```python
from build123d import *

# Parameters (mm, degrees)
BOSS_EXTRUDE1_DEPTH = 28.575
CHAMFER1_SIZE       = 6.35
SKETCH3_R           = 1.905
CUT_EXTRUDE1_DEPTH  = 62.321512782
FILLET1_R           = 3.175
CUT_EXTRUDE4_START  = -6.35
CUT_EXTRUDE4_DEPTH  = 6.35
FILLET3_R           = 1.5875
FILLET5_R           = 1.5875


with BuildPart() as part:
    # Sketch2 → Boss-Extrude1 (new body)
    with BuildSketch(Plane.XY):
        with BuildLine():
            Line((0, 0), (19.056686619, 0))
            ThreePointArc((19.056686619, 0), (7.311521051, 25.4), (19.056686619, 50.8))
            Line((19.056686619, 50.8), (0, 50.8))
            Line((0, 50.8), (0, 0))
        make_face()
    extrude(amount=BOSS_EXTRUDE1_DEPTH)

    # Chamfer1
    chamfer1_edges = [part.edges().sort_by_distance(p)[0] for p in [
        (0, 0, 14.2875),
    ]]
    chamfer(chamfer1_edges, length=CHAMFER1_SIZE)

    # Sketch3 → Cut-Extrude1 (cut, through all)
    with BuildSketch(Plane.XY.offset(28.575)):
        with Locations((5.55625, 45.24375)):
            Circle(SKETCH3_R)
        with Locations((5.55625, 8.651474106)):
            Circle(SKETCH3_R)
    extrude(amount=-CUT_EXTRUDE1_DEPTH, mode=Mode.SUBTRACT)

    # Fillet1
    fillet1_edges = [part.edges().sort_by_distance(p)[0] for p in [
        (0, 50.8, 14.2875),
        (6.35, 0, 14.2875),
        (0, 6.35, 14.2875),
    ]]
    fillet(fillet1_edges, radius=FILLET1_R)

    # Sketch6 → Cut-Extrude4 (cut)
    with BuildSketch(Plane.XY.offset(28.575).offset(CUT_EXTRUDE4_START)):
        with BuildLine():
            Line((5.55625, 49.2125), (17.317631251, 49.2125))
            ThreePointArc((17.317631251, 49.2125), (14.028288765, 45.468022294), (11.333951868, 41.275))
            Line((11.333951868, 41.275), (5.55625, 41.275))
            ThreePointArc((5.55625, 41.275), (1.5875, 45.24375), (5.55625, 49.2125))
        make_face()
        with BuildLine():
            Line((5.55625, 12.620224106), (9.858336838, 12.620224106))
            ThreePointArc((9.858336838, 12.620224106), (11.918918568, 8.489348991), (14.530380471, 4.682724106))
            Line((14.530380471, 4.682724106), (5.55625, 4.682724106))
            ThreePointArc((5.55625, 4.682724106), (1.5875, 8.651474106), (5.55625, 12.620224106))
        make_face()
    extrude(amount=CUT_EXTRUDE4_DEPTH, mode=Mode.SUBTRACT)

    # Fillet3
    fillet3_edges = [part.edges().sort_by_distance(p)[0] for p in [
        (19.056686619, 0, 14.2875),
        (19.056686619, 50.8, 14.2875),
    ]]
    fillet(fillet3_edges, radius=FILLET3_R)

    # Fillet5
    fillet5_edges = [part.edges().sort_by_distance(p)[0] for p in [
        (11.333951868, 41.275, 25.4),
        (9.858336838, 12.620224106, 25.4),
    ]]
    fillet(fillet5_edges, radius=FILLET5_R)


solid = part.part
```
Geometry: final body of the model. Coordinates: model frame, mm. A direction names the side the tool comes from. Coordinates: 2 decimals unless noted, no trailing zeros. Order: outer loops, then holes, each group sorted by start corner. A loop starts at its lowest first (then second) coordinate and runs counter-clockwise, first axis right, second up. Notation, with made-up numbers: M 23,55.25 L 82,55.25 A6 cw 82,59.25 Z; hole C 28.5,79 d9. An arc over 180 degrees is marked long. Answer in a Markdown table with one row per item. Add a question column.
Q1. Section query B-B on z = 8.25. Count the separate pieces of the cut face and the enclosed holes in it, and give its area (3 significant figures).
Q2. Contact query for flat-ended pins moving along their axis: P1, Ø5, axis at x = 5.56, y = 8.65, coming from the +Z side (3 decimals); P2, Ø8, axis at y = 10, z = 15.5, coming from the +X side; P3, Ø6, axis at x = 13, y = 40.5, coming from the +Z side (3 decimals); P4, Ø1.6, axis at x = 6.5, z = 25.5, coming from the -Y side. Output: stop coordinate, or through.
Q3. Reachability of faces 5 (the cylindrical face through (8.87, 13.3, 25.44)), 6 (the cylindrical face through (6.466, 0.235, 14.488)) from +Z, -Z, +X, -X, +Y, -Y: full face, straight path, thin tool, end or side. Return the list, or none.
Q4. Line query: L1, parallel to Y at x = 12, z = 27; L2, parallel to Y at x = 7.25, z = 2; L3, parallel to Y at x = 3.25, z = 27. Output: solid intervals per line, ascending.
Q5. Section query D-D on y = 21. Return the cut outline in (x, z) (3 decimals), and give its area (3 significant figures).
Q6. Section query A-A on x = 14. Return the cut outline in (y, z) (1 decimal), and give its area (3 significant figures).
Q7. Mould query, pull axis X, two halves, no side actions, for faces 1 (the cylindrical face through (1.59, 8.56, 25.36)), 2 (the cylindrical face through (0.91, 49.85, 14.49)), 3 (the cylindrical face through (5.1, 6.8, 11.3)), 4 (the flat face through (11, 49.212, 25)). Classes: released by +X, released by -X, zero draft, split by the parting line, or undercut.
Completed:
| question | item | result |
|---|---|---|
| 1 | separate pieces | 1 |
| 1 | enclosed holes | 2 |
| 1 | area | 502 mm2 |
| 2 | P1 | stops at z = 22.225 |
| 2 | P2 | stops at x = 13.54 |
| 2 | P3 | stops at z = 28.575 |
| 2 | P4 | stops at y = 0.02 |
| 3 | face 5 | +Z, +X |
| 3 | face 6 | +Z, -Z, -X, -Y |
| 4 | L1 | y = 0 to 4.68, 49.21 to 50.8 |
| 4 | L2 | y = 0.03 to 7.78, 9.52 to 44.37, 46.12 to 50.8 |
| 4 | L3 | y = 3.1 to 5.42, 11.88 to 42.01, 48.47 to 50.8 |
| 5 | outline | M 0,0 L 7.603,0 L 7.603,28.575 L 0,28.575 Z |
| 5 | area | 217 mm2 |
| 6 | outline | M 0,0 L 5.4,0 L 5.4,22.2 L 4.7,22.2 L 4.7,28.6 L 0,28.6 Z; M 45.4,0 L 50.8,0 L 50.8,28.6 L 49.2,28.6 L 49.2,22.2 L 45.4,22.2 Z |
| 6 | area | 278 mm2 |
| 7 | face 1 | released by +X |
| 7 | face 2 | released by -X |
| 7 | face 3 | undercut |
| 7 | face 4 | zero draft |
